Design review of the part built by this model. Coordinates are the model's own, in mm. Face numbers are marked on the shaded views. Coordinates: 2 decimals unless noted, no trailing zeros. Loops run counter-clockwise (first coordinate to the right, second up) from the corner with the lowest first, then second, coordinate; pieces in that order, holes last. Notation, with made-up numbers: M 32.5,-27.75 L 39.5,-27.75 A16 cw 39.5,3.25 Z; hole C 70.25,50.5 d8. An arc over 180 degrees is marked long. Put each result on its own line as item: value. Start each with the question number.
(1) Take a section at B-B, the plane x = 4.3. Give the boundary of the cut face in (y, z) (3 decimals).
(2) Take a section at D-D, the plane y = 41. Give the boundary of the cut face in (x, z).
(3) Clearance check with flat-ended pins moving along their axes: pin 1 (3 mm diameter, centred on x = 4.5, z = -44.5, fed in from +Y); pin 2 (11.5 mm diameter, centred on y = 18.5, z = -36.5, fed in from +X); pin 3 (2 mm diameter, centred on x = 8.5, z = -44, fed in from -Y). State where each tip first meets the part, or that it passes through.
(4) Take a section at C-C, the plane y = 22.5. Give the boundary of the cut face in (x, z), then the cut area to 3 significant figures.
(5) For probe 1 along Z at (x, y) = (8.1, 25.4); probe 2 along Y at (x, z) = (7.05, -38.1); probe 3 along Z at (x, y) = (6.2, 30), list the stretches that pass through material, from the lowest coordinate up. Write a range as [from, to].
(6) Take a section at A-A, the plane z = -38.1. Give the boundary of the cut face in (x, y).
(7) The part is to be moulded in two halves that separate along Z. For the marked faces 1, 2, 3 and 4, say which applies: +Z half, -Z half, draft (parallel to the pull), parting line (faces both ways), or undercut.
Autodesk Inventor part; units mm, degrees
ref_plane "YZ Plane" through (0, 0, 0) normal (1, 0, 0) x (0, 1, 0)
ref_plane "XZ Plane" through (0, 0, 0) normal (0, 1, 0) x (-1, 0, 0)
ref_plane "XY Plane" through (0, 0, 0) normal (0, 0, 1) x (1, 0, 0)
sketch "Sketch1" plane through (0, 0, 0) normal (0, 1, 0) x (-1, 0, 0)
  line L0 (0, 0) -> (-20.32, 0)
  line L1 (-20.32, 0) -> (-20.32, -76.2)
  line L2 (-20.32, -76.2) -> (0, -76.2)
  line L3 (0, -76.2) -> (0, 0)
  dimension "d0" = 20.32
  dimension "d1" = 76.2
extrude "Extrusion1" add sketch "Sketch1" along normal blind 7.62
sketch "Sketch2" plane through (0, 7.62, 0) normal (0, 1, 0) x (1, 0, 0)
  line L0 (0, 0) -> (0, 12.7)
  line L1 (0, 12.7) -> (20.32, 12.7)
  line L2 (20.32, 12.7) -> (20.32, 63.5)
  line L3 (20.32, 63.5) -> (0, 63.5)
  line L4 (0, 63.5) -> (0, 12.7)
  dimension "d4" = 12.7
  dimension "d5" = 20.32
  dimension "d6" = 50.8
extrude "Extrusion2" add sketch "Sketch2" along normal blind 43.18
sketch "Sketch3" plane through (20.32, 0, 0) normal (1, 0, 0) x (0, 0, -1)
  line L0 (12.7, 50.8) -> (63.5, 50.8)
  line L1 (38.1, 50.8) -> (38.1, 25.4)
  circle A0 centre (38.1, 25.4) radius 19.05
  point P0 (0, 0)
  dimension "d9" = 25.4
  dimension "d10" = 38.1
extrude "Extrusion3" cut sketch "Sketch3" against normal blind 15.24
fillet "Fillet1" radius 25.4 2 edges at (10.16, 50.8, -63.5) (10.16, 50.8, -12.7)
sketch "Sketch6" plane through (0, 7.62, 0) normal (0, 1, 0) x (1, 0, 0)
  line L0 (0, 0) -> (20.32, 0)
  line L1 (10.16, 0) -> (10.16, 6.35)
  line L2 (20.32, 76.2) -> (0, 76.2)
  line L3 (10.16, 76.2) -> (10.16, 69.85)
  dimension "d20" = 6.35
  dimension "d21" = 6.35
fillet "Fillet2" radius 25.4 2 edges at (10.16, 7.62, -63.5) (10.16, 7.62, -12.7)
hole "Hole1" at (10.16, 7.62, -6.35) at (10.16, 7.62, -69.85) direction (0, -1, 0) diameter 5.08 end through all counterbore diameter 10.16 counterbore depth 3.81
sketch "Sketch7" plane through (10.16, 7.62, -6.35) normal (0, -1, 0) x (1, 0, 0)
  circle A0 centre (0, 0) radius 5.08
  circle A1 centre (0, -63.5) radius 2.54
  line L0 (-2.54, -63.5) -> (0, -63.5)
  circle A2 centre (0, -63.5) radius 5.08
  point P0 (-10.16, 6.35)
  dimension "d30" = 10.16
  dimension "d31" = 10.16
extrude "Extrusion5" cut sketch "Sketch7" against normal blind 15.24 contours A0 | A1 | A2
sketch "Sketch10" plane through (5.08, 25.4, -38.1) normal (1, 0, 0) x (0, 0, -1)
  line L0 (0, 0) -> (0, 6.35)
  circle A0 centre (0, 6.35) radius 6.35
  line L1 (0, 0) -> (-7.874, 13.6382)
  line L2 (0, 0) -> (15.748, 0) construction
  line L3 (0, 0) -> (7.874, 13.6382)
  line L4 (0, 0) -> (15.748, 0) construction
  circle A1 centre (-7.874, 13.6382) radius 1.651
  circle A2 centre (7.874, 13.6382) radius 1.651
  point P0 (-38.1, -25.4)
  dimension "d65" = 6.35
  dimension "d85" = 15.748
  dimension "d86" = 120
  dimension "d87" = 15.748
  dimension "d88" = 60
  dimension "d89" = 3.302
  dimension "d90" = 3.302
extrude "Extrusion8" cut sketch "Sketch10" against normal blind 25.4 contours L3 A0 | A0 L1 | L1 A0 L3
sketch "Sketch13" plane through (5.08, 25.4, -38.1) normal (1, 0, 0) x (0, 0, -1)
  circle A0 centre (0, 6.35) radius 6.35
  point P0 (-38.1, -25.4)
  point P1 (0, 0)
pattern_circular "Circular Pattern3" count 6 over 360 about axis through (5.08, 25.4, -38.1) along (1, 0, 0) of "Extrusion8"
sketch "Sketch14" plane through (5.08, 25.4, -38.1) normal (1, 0, 0) x (0, 0, -1)
  circle A0 centre (0, 0) radius 20.2652
  circle A1 centre (0, 0) radius 51.9893
  point P0 (-38.1, -25.4)
extrude "Extrusion10" cut sketch "Sketch14" against normal mid plane 50.8
sketch "Sketch15" plane through (20.32, 25.4, -38.1) normal (1, 0, 0) x (0, 0, -1)
  circle A0 centre (0, 0) radius 23.435
  point P0 (-38.1, -25.4)
extrude "Extrusion11" cut sketch "Sketch15" against normal blind 11.43
sketch "Sketch16" plane through (0, 25.4, -38.1) normal (-1, 0, 0) x (0, 0, 1)
  circle A0 centre (0, 0) radius 24.6265
  point P0 (38.1, -25.4)
extrude "Extrusion12" cut sketch "Sketch16" against normal blind 3.81
properties part number "Motor Mount V2"
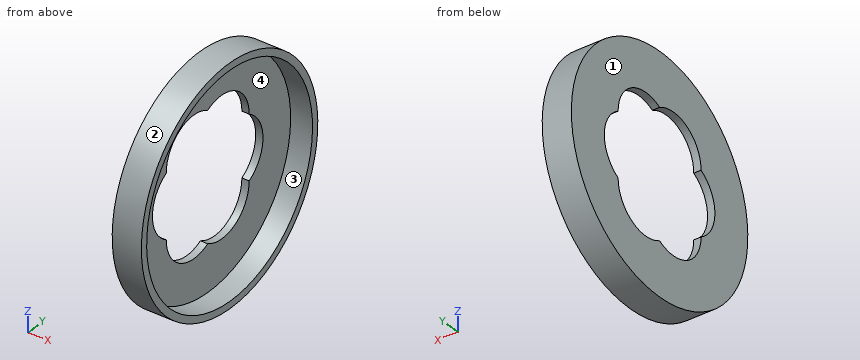
Computed values:
1. outline: C 25.4,-38.1 d40.53; hole M 15.875,-43.599 A6.35 ccw 25.4,-49.099 A6.35 ccw 34.925,-43.599 A6.35 ccw 34.925,-32.601 A6.35 ccw 25.4,-27.101 A6.35 ccw 15.875,-32.601 A6.35 ccw Z
2. outline: M 3.81,-51.04 L 8.89,-51.04 L 8.89,-49.03 L 5.08,-49.03 L 5.08,-27.17 L 8.89,-27.17 L 8.89,-25.16 L 3.81,-25.16 Z
3. pin 1: stops at y = 45.06
3. pin 2: stops at x = 5.08
3. pin 3: stops at y = 5.74
4. outline: M 3.81,-58.16 L 8.89,-58.16 L 8.89,-56.93 L 5.08,-56.93 L 5.08,-49.94 L 3.81,-49.94 Z; M 3.81,-26.26 L 5.08,-26.26 L 5.08,-19.27 L 8.89,-19.27 L 8.89,-18.04 L 3.81,-18.04 Z
4. area: 30.2 mm^2
5. probe 1: z = [-58.37, -57.15], [-19.05, -17.83]
5. probe 2: y = [5.13, 6.35], [44.45, 45.67]
5. probe 3: z = [-57.84, -56.59], [-19.61, -18.36]
6. outline: M 3.81,5.13 L 8.89,5.13 L 8.89,6.35 L 5.08,6.35 L 5.08,12.7 L 3.81,12.7 Z; M 3.81,38.1 L 5.08,38.1 L 5.08,44.45 L 8.89,44.45 L 8.89,45.67 L 3.81,45.67 Z
7. face 1: draft
7. face 2: parting line
7. face 3: undercut
7. face 4: undercut
